from build123d import *


with BuildPart() as part:
    # Esquisse1 → Révolution1 (revolve)
    with BuildSketch(Plane(origin=(0, 0, 0), x_dir=(1, 0, 0), z_dir=(0, 1, 0)), mode=Mode.PRIVATE) as r_volution1_sk:
        with BuildLine():
            Line((29.9, 17.303746522), (29.9, 17.713746522))
            Line((29.9, 17.713746522), (0, 17.713746522))
            Line((0, 17.713746522), (0, 17.052896028))
            Line((0, 17.052896028), (1, 17.052896028))
            Line((1, 17.052896028), (1, 8.013746522))
            Line((1, 8.013746522), (7.558685201, 8.013746522))
            Line((7.558685201, 8.013746522), (7.558685201, 14.313746522))
            Line((7.558685201, 14.313746522), (29.9, 14.313746522))
            Line((29.9, 14.313746522), (29.9, 14.723746522))
            ThreePointArc((29.9, 14.723746522), (31.19, 16.013746522), (29.9, 17.303746522))
        make_face()
    revolve(r_volution1_sk.sketch.rotate(Axis((0, 0, -20.028610737), (0, 0, 1)), 180), axis=Axis((0, 0, -20.028610737), (0, 0, 1)))


solid = part.part
Part model, mm, in its own coordinate system. A direction names the side the tool comes from. Coordinates: 2 decimals unless noted, no trailing zeros. Loops run counter-clockwise (first coordinate to the right, second up) from the corner with the lowest first, then second, coordinate; pieces in that order, holes last. Notation, with made-up numbers: M 18.5,25.5 L 22.5,25.5 A25 ccw 22.5,63.5 Z; hole C -20,86.5 d8. An arc over 180 degrees is marked long. Use a Markdown table: item, result. Add a question column.
Q1. Probe L1, parallel to Y at x = 0, z = -11.5; L2, parallel to Y at x = 0, z = -14.5; L3, parallel to Z at x = 6, y = -29. List the from-to ranges inside material, lowest first.
Q2. Which spindle directions (+Z, -Z, +X, -X, +Y, -Y) get a long thin tool onto all of the face, cutting with end or side? Do faces 4 (the cylindrical face through (-13.797, 26.526, -17.512)), 5 (the cylindrical face through (1.64, 7.38, -11.21)), 6 (the flat face through (0, 2, -8.014)). Say none if no direction does.
Q3. Cut at B-B (z = -9.75). Write the cut outline in (x, y), and give its area (3 significant figures).
Q4. Pin check, flat tips, straight feed: P1, Ø1.5, axis at x = 24.5, z = -15, coming from the +Y side; P2, Ø4, axis at x = 16.5, y = 6.5, coming from the +Z side; P3, Ø5, axis at y = 20, z = -13, coming from the -X side. Stop position of each tip, or through.
Q5. Cut at D-D (z = -16). Write the cut outline in (x, y), and give its area (3 significant figures).
Q6. Mould opens along X. For faces 1 (the flat face through (0, 0, -17.053)), 2 (the cylindrical face through (-13.797, 26.526, -14.522)), 3 (the flat face through (6, 6, -14.314)) say: +X half, -X half, draft (parallel to the pull), parting line (faces both ways), or undercut.
Q7. Cut at A-A (x = 0). Write the cut outline in (y, z).
Worked out:
| question | item | result |
|---|---|---|
| 1 | L1 | y = -7.56 to -1, 1 to 7.56 |
| 1 | L2 | y = -29.9 to -1, 1 to 29.9 |
| 1 | L3 | z = -17.71 to -14.31 |
| 2 | face 4 | -Z |
| 2 | face 5 | +Z |
| 2 | face 6 | +Z, +X, -X, +Y, -Y |
| 3 | outline | C 0,0 d15.12; hole C 0,0 d2 |
| 3 | area | 176 mm2 |
| 4 | P1 | stops at y = 19.84 |
| 4 | P2 | stops at z = -14.31 |
| 4 | P3 | stops at x = -24.53 |
| 5 | outline | C 0,0 d62.38; hole C 0,0 d2 |
| 5 | area | 3,050 mm2 |
| 6 | face 1 | undercut |
| 6 | face 2 | parting line |
| 6 | face 3 | draft |
| 7 | outline | M -29.9,-17.71 L 29.9,-17.71 L 29.9,-17.3 A1.29 ccw 29.9,-14.72 L 29.9,-14.31 L 7.56,-14.31 L 7.56,-8.01 L 1,-8.01 L 1,-17.05 L -1,-17.05 L -1,-8.01 L -7.56,-8.01 L -7.56,-14.31 L -29.9,-14.31 L -29.9,-14.72 A1.29 ccw -29.9,-17.3 Z |
